from build123d import *

# Parameters (mm, degrees)
CROQUIS1_R              = 2.034348523
CROQUIS1_R_2            = 3
SALIENTE_EXTRUIR1_DEPTH = 2
SALIENTE_EXTRUIR2_DEPTH = 2
MATRIZC1_COUNT          = 8
MATRIZC1_ANGLE          = 128
CROQUIS4_R              = 1.53
CORTAR_EXTRUIR1_DEPTH   = 10


with BuildPart() as part:
    # Croquis1 → Saliente-Extruir1 (new body)
    with BuildSketch(Plane(origin=(0, 0, 0), x_dir=(1, 0, 0), z_dir=(0, 1, 0))):
        with BuildLine():
            Line((-5, -10.339498295), (-5, -30))
            ThreePointArc((-5, -30), (0, -35), (5, -30))
            Line((5, -30), (5, -10.339498295))
            ThreePointArc((5, -10.339498295), (0, 11.485), (-5, -10.339498295))
        make_face()
        with Locations((0, -30)):
            Circle(CROQUIS1_R, mode=Mode.SUBTRACT)
        Circle(CROQUIS1_R_2, mode=Mode.SUBTRACT)
    extrude(amount=SALIENTE_EXTRUIR1_DEPTH)

    # Croquis3 → Saliente-Extruir2 (add)
    with BuildSketch(Plane(origin=(0, 0, 0), x_dir=(1, 0, 0), z_dir=(0, 1, 0))):
        with BuildLine():
            Line((1.120443051, 12.967936283), (0.853363456, 11.45325263))
            ThreePointArc((0.853363456, 11.45325263), (1.994349321, 11.310517043), (3.115343764, 11.054404472))
            Line((3.115343764, 11.054404472), (3.382423359, 12.569088125))
            Line((3.382423359, 12.569088125), (3.089673258, 14.215613789))
            ThreePointArc((3.089673258, 14.215613789), (2.526146865, 14.326490787), (1.958683104, 14.415037868))
            Line((1.958683104, 14.415037868), (1.120443051, 12.967936283))
        make_face()
    saliente_extruir2 = extrude(amount=SALIENTE_EXTRUIR2_DEPTH)

    # MatrizC1: Saliente-Extruir2 ×8 about axis
    matrizc1_axis = Axis((0, 0, 0), (0, 1, 0))
    for i in range(1, MATRIZC1_COUNT):
        add(saliente_extruir2.rotate(matrizc1_axis, i * MATRIZC1_ANGLE / (MATRIZC1_COUNT - 1)))

    # Croquis4 → Cortar-Extruir1 (cut)
    with BuildSketch(Plane.XZ):
        with Locations((0.559982615, -7.634490453)):
            Circle(CROQUIS4_R)
        with Locations((0, 7.655)):
            Circle(CROQUIS4_R)
    extrude(amount=-CORTAR_EXTRUIR1_DEPTH, mode=Mode.SUBTRACT)


solid = part.part
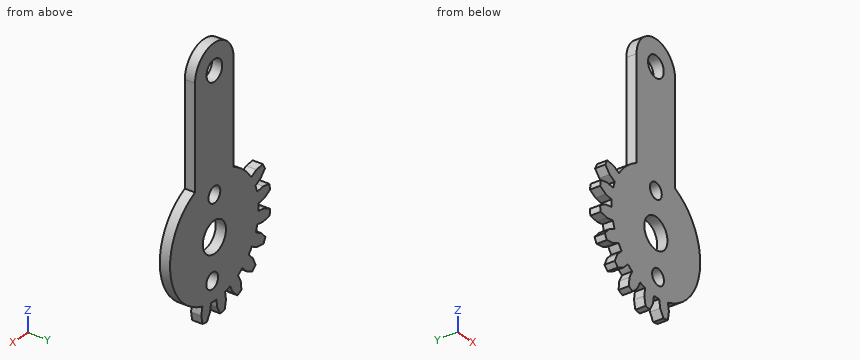
Check sheet for the modelled part. Datum: model origin and axes. Units: mm. Give positions to 0.01 mm unless a question says otherwise; leave off trailing zeros. Loops run counter-clockwise (first coordinate to the right, second up) from the corner with the lowest first, then second, coordinate; pieces in that order, holes last. Notation, with made-up numbers: M -4,-21 L 2,-21 A21 cw 2,11 Z; hole C 58,-26 d7. An arc over 180 degrees is marked long. Use a Markdown table: item, result. Add a question column.
Q1. Sectioned sample at C-C, the plane z = 24.5. Record the cut outline in (x, y).
Q2. Sectioned sample at A-A, the plane z = 0. Record the cut outline in (x, y) (3 decimals), then the cut area to 3 significant figures.
Q3. Sectioned sample at D-D, the plane y = 1.5. Give the number of separate pieces and of enclosed holes in the cut face, then the cut area to 3 significant figures.
Q4. Go/stop test with flat-tipped pins: pin 1 (8 mm diameter, centred on x = -8.5, z = -5, fed in from -Y); pin 2 (0.6 mm diameter, centred on y = 0.5, z = 19, fed in from -X); pin 3 (1 mm diameter, centred on x = -5, y = 0.5, fed in from +Z). Record where each tip stops, or that it passes through.
Q5. Sectioned sample at B-B, the plane x = 0. Record the cut outline in (y, z) (3 decimals), then the cut area to 3 significant figures.
Q6. Scan lines: line 1 along Z through (x, y) = (1.25, 0.9); line 2 along X through (y, z) = (1.85, 30); line 3 along X through (y, z) = (0.5, 0) (3 decimals). Record each from-to range of solid material in increasing order. Write a range as [from, to].
Verdict:
| question | item | result |
|---|---|---|
| 1 | outline | M -5,0 L 5,0 L 5,2 L -5,2 Z |
| 2 | outline | M -11.485,0 L -3,0 L -3,2 L -11.485,2 Z; M 3,0 L 11.485,0 L 11.485,2 L 3,2 Z |
| 2 | area | 33.9 mm^2 |
| 3 | separate pieces | 1 |
| 3 | enclosed holes | 4 |
| 3 | area | 636 mm^2 |
| 4 | pin 1 | y = 0 |
| 4 | pin 2 | x = -5 |
| 4 | pin 3 | z = 32.18 |
| 5 | outline | M 0,-11.485 L 2,-11.485 L 2,-9.058 L 0,-9.058 Z; M 0,-6.211 L 2,-6.211 L 2,-3 L 0,-3 Z; M 0,3 L 2,3 L 2,6.125 L 0,6.125 Z; M 0,9.185 L 2,9.185 L 2,27.966 L 0,27.966 Z; M 0,32.034 L 2,32.034 L 2,35 L 0,35 Z |
| 5 | area | 61.0 mm^2 |
| 6 | line 1 | [-13.19, -9], [-6.27, -2.73], [2.73, 6.77], [8.54, 28.39], [31.61, 34.84] |
| 6 | line 2 | [-5, -2.03], [2.03, 5] |
| 6 | line 3 | [-11.485, -3], [3, 11.485] |
